from build123d import *

# Parameters (mm, degrees)
SKETCH2_R           = 15
BOSS_EXTRUDE1_DEPTH = 4
SKETCH3_W           = 15
SKETCH3_H           = 17
BOSS_EXTRUDE2_DEPTH = 4
SKETCH4_R           = 1.6
CUT_EXTRUDE1_DEPTH  = 23.671568098
SKETCH5_R           = 2.95
CUT_EXTRUDE2_DEPTH  = 6.1


with BuildPart() as part:
    # Sketch2 → Boss-Extrude1 (new body)
    with BuildSketch(Plane(origin=(0, 0, 0), x_dir=(1, 0, 0), z_dir=(0, 1, 0))):
        with Locations(Location((0, 0, 0), (0, 0, 270))):
            Circle(SKETCH2_R)
    extrude(amount=BOSS_EXTRUDE1_DEPTH)

    # Sketch3 → Boss-Extrude2 (add)
    with BuildSketch(Plane(origin=(0, 4, 0), x_dir=(1, 0, 0), z_dir=(0, 1, 0))):
        Rectangle(SKETCH3_W, SKETCH3_H)
    extrude(amount=BOSS_EXTRUDE2_DEPTH)

    # Sketch4 → Cut-Extrude1 (cut, through all)
    with BuildSketch(Plane(origin=(0, 8, 0), x_dir=(1, 0, 0), z_dir=(0, 1, 0))):
        with Locations(Location((0, 3.5, 0), (0, 0, 270))):
            Circle(SKETCH4_R)
        with Locations(Location((0, -3.5, 0), (0, 0, 90))):
            Circle(SKETCH4_R)
    extrude(amount=-CUT_EXTRUDE1_DEPTH, mode=Mode.SUBTRACT)

    # Sketch5 → Cut-Extrude2 (cut)
    with BuildSketch(Plane.XZ):
        with Locations(Location((0, 3.5, 0), (0, 0, 270))):
            Circle(SKETCH5_R)
        with Locations(Location((0, -3.5, 0), (0, 0, 90))):
            Circle(SKETCH5_R)
    extrude(amount=-CUT_EXTRUDE2_DEPTH, mode=Mode.SUBTRACT)


solid = part.part
Model file for the job. Use its own axes, mm. A direction names the side the tool comes from. Give positions to 0.01 mm unless a question says otherwise; leave off trailing zeros. Loops run counter-clockwise (first coordinate to the right, second up) from the corner with the lowest first, then second, coordinate; pieces in that order, holes last. Notation, with made-up numbers: (19.5, -15) -> (41.5, -15) arc R16 ccw to (41.5, 7) -> close; hole circle Ø4 at (-34, -8). An arc over 180 degrees is marked (long way). Use a Markdown table: item, result. Add a question column.
(1) Slice it at C-C on y = 6.5. List the corners of the cut face in (x, z).
(2) Drop flat-ended pins along their axis: pin 1 Ø3 at (x, z) = (-1, 2.5) entering from -Y; pin 2 Ø4 at (y, z) = (5, 6.5) entering from -X; pin 3 Ø1 at (x, y) = (-2.5, 2.5) entering from +Z. Give the stop position or say it passes through.
(3) Wall check: line 1 along X through (y, z) = (7.15, -3.5); line 2 along X through (y, z) = (5, 3.5); line 3 along Y through (x, z) = (-6.5, -9.25). Give the ranges that are in metal, low to high.
(4) Slice it at D-D on z = -3.5. List the corners of the cut face in (x, y), and give its area (3 significant figures).
(5) Tool access for faces 1 (the flat face through (0, 6, -8.5)), 2 (the flat face through (0, 6, 8.5)), 3 (the flat face through (1, 6.1, -2)): list every direction of +Z, -Z, +X, -X, +Y, -Y with a clear straight run to the whole face (end or side of a thin tool).
(6) Mould opens along X. For faces 4 (the flat face through (-10, 4, 0)), 5 (the cylindrical face through (0.66, 1.972, -14.985)), 6 (the cylindrical face through (-1.13, 3.007, 0.775)), 7 (the cylindrical face through (0.61, 7.06, 2.02)) say: +X half, -X half, draft (parallel to the pull), parting line (faces both ways), or undercut.
(7) Slice it at A-A on x = 0. List the corners of the cut face in (y, z).
(8) Slice it at B-B on z = 0. List the corners of the cut face in (x, y).
Filled sheet:
| question | item | result |
|---|---|---|
| 1 | outline | (-7.5, -8.5) -> (7.5, -8.5) -> (7.5, 8.5) -> (-7.5, 8.5) -> close; hole circle Ø3.2 at (0, -3.5); hole circle Ø3.2 at (0, 3.5) |
| 2 | pin 1 | y = 6.1 |
| 2 | pin 2 | x = -14.22 |
| 2 | pin 3 | z = 14.87 |
| 3 | line 1 | -7.5 to -1.6, 1.6 to 7.5 |
| 3 | line 2 | -7.5 to -2.95, 2.95 to 7.5 |
| 3 | line 3 | 0 to 4 |
| 4 | outline | (-14.59, 0) -> (-2.95, 0) -> (-2.95, 6.1) -> (-1.6, 6.1) -> (-1.6, 8) -> (-7.5, 8) -> (-7.5, 4) -> (-14.59, 4) -> close; (1.6, 6.1) -> (2.95, 6.1) -> (2.95, 0) -> (14.59, 0) -> (14.59, 4) -> (7.5, 4) -> (7.5, 8) -> (1.6, 8) -> close |
| 4 | area | 135 mm2 |
| 5 | face 1 | -Z, +X, -X, +Y |
| 5 | face 2 | +Z, +X, -X, +Y |
| 5 | face 3 | -Y |
| 6 | face 4 | draft |
| 6 | face 5 | parting line |
| 6 | face 6 | undercut |
| 6 | face 7 | undercut |
| 7 | outline | (0, -15) -> (4, -15) -> (4, -8.5) -> (8, -8.5) -> (8, -5.1) -> (6.1, -5.1) -> (6.1, -6.45) -> (0, -6.45) -> close; (0, -0.55) -> (6.1, -0.55) -> (6.1, -1.9) -> (8, -1.9) -> (8, 1.9) -> (6.1, 1.9) -> (6.1, 0.55) -> (0, 0.55) -> close; (0, 6.45) -> (6.1, 6.45) -> (6.1, 5.1) -> (8, 5.1) -> (8, 8.5) -> (4, 8.5) -> (4, 15) -> (0, 15) -> close |
| 8 | outline | (-15, 0) -> (15, 0) -> (15, 4) -> (7.5, 4) -> (7.5, 8) -> (-7.5, 8) -> (-7.5, 4) -> (-15, 4) -> close |
